Could you check a few things on this model? Use its own coordinates, in mm. A direction names the side the tool comes from. Give positions to 0.01 mm unless a question says otherwise; leave off trailing zeros. Loops run counter-clockwise (first coordinate to the right, second up) from the corner with the lowest first, then second, coordinate; pieces in that order, holes last. Notation, with made-up numbers: (73, -26.5) -> (83, -26.5) arc R21 cw to (83, 2.5) -> close; hole circle Ø5 at (8.25, 31). An arc over 180 degrees is marked (long way). Write item = value, one per line. Start each with the question number.
1) I'm going to push flat-ended pins straight in: pin 1 Ø12 at (x, y) = (-61, 43) entering from +Z; pin 2 Ø12 at (x, z) = (-46.5, 20) entering from +Y; pin 3 Ø2 at (x, y) = (-22, 42.5) entering from +Z. Where does each tip first touch, or does it pass through?
2) I want a section at C-C (x = -42.5). List the corners of the cut face in (y, z) for me.
3) I need wall thicknesses on probe 1 along X at (y, z) = (49.5, 10); probe 2 along Z at (x, y) = (-44, 36); probe 3 along Y at (x, z) = (-41, 29). Which ranges of each line are inside material? Lowest first, please. Write a range as from..to.
4) I want a section at B-B (z = 31). List the corners of the cut face in (x, y) for me.
5) On a 3-axis mill with a long thin cutter (end or side, diameter ignored), from which of +Z, -Z, +X, -X, +Y, -Y can I reach the whole of each face in a straight line? I mean faces 1 (the face through (-53.23, 33.17, 22.19)), 2 (the face through (-75, 18, 18)). Say none if no direction works.
6) I want a section at A-A (y = 34). List the corners of the cut face in (x, z) for me, and give its area (3 significant figures).
from build123d import *

# Parameters (mm, degrees)
EXTRUDE1_DEPTH = 75
EXTRUDE2_DEPTH = 75


with BuildPart() as part:
    # Sketch1 → Extrude1 (new body)
    with BuildSketch(Plane(origin=(0, 0, 0), x_dir=(1, 0, 0), z_dir=(0, 1, 0))):
        Polygon((0, 0), (0, -45), (-20, -45), (-40, 0), align=None)
    extrude(amount=EXTRUDE1_DEPTH)

    # Sketch2 → Extrude2 (add)
    with BuildSketch(Plane(origin=(0, 0, 0), x_dir=(0, 0, -1), z_dir=(1, 0, 0))):
        Polygon((-45, 20), (-45, 0), (0, 0), (0, 45.980762114), align=None)
    extrude(amount=-EXTRUDE2_DEPTH)


solid = part.part
Answer list:
q1.pin_1 = 15.56
q1.pin_2 = 37.9
q1.pin_3 = 42.75
q2.outline = (0, 0) -> (45.98, 0) -> (20, 45) -> (0, 45) -> close
q3.probe_1 = -35.56..0
q3.probe_2 = 0..17.29
q3.probe_3 = 0..29.24
q4.outline = (-75, 0) -> (0, 0) -> (0, 75) -> (-26.22, 75) -> (-26.22, 28.08) -> (-75, 28.08) -> close
q5.face_1 = +Z, -X, +Y
q5.face_2 = +Z, -Z, -X, +Y, -Y
q6.outline = (-75, 0) -> (0, 0) -> (0, 45) -> (-20, 45) -> (-30.78, 20.75) -> (-75, 20.75) -> close
q6.area = 2,170 mm^2
